Geometry: final body of the model. Coordinates: model frame, mm. A direction names the side the tool comes from. Round coordinates to 2 decimals unless told otherwise and drop trailing zeros. Loops run counter-clockwise (first coordinate to the right, second up) from the corner with the lowest first, then second, coordinate; pieces in that order, holes last. Notation, with made-up numbers: M -8.5,43.25 L 1.5,43.25 A27 ccw 1.5,75.25 Z; hole C 69,4.25 d5. An arc over 180 degrees is marked long. Return JSON: item names as keys, results as strings.
from build123d import *

# Parameters (mm, degrees)
BASPROSKE_W         = 5
BASPROSKE_H         = 11
TOOTHCUT_DEPTH      = 17.340134638
TEETHCUTS_COUNT     = 20
BORSKE_R            = 1.5
BORE_DEPTH          = 50.0000508
SKETCH_1_R          = 6
EXTRUDE_1_DEPTH     = 6
CUT_EXTRUDE_1_DEPTH = 14
SKETCH_3_R          = 2.7
CUT_EXTRUDE_2_DEPTH = 3


with BuildPart() as part:
    # BasProSke → Base-Revolve (revolve)
    with BuildSketch(Plane(origin=(0, 0, 0), x_dir=(1, 0, 0), z_dir=(0, 1, 0)), mode=Mode.PRIVATE) as base_revolve_sk:
        with Locations((2.5, 5.5)):
            Rectangle(BASPROSKE_W, BASPROSKE_H)
    revolve(base_revolve_sk.sketch.rotate(Axis((-10, 0, 0), (1, 0, 0)), 180), axis=Axis((-10, 0, 0), (1, 0, 0)))

    # TooCutSke → ToothCut (cut, through all)
    with BuildSketch(Plane(origin=(0, 0, 0), x_dir=(0, 0, -1), z_dir=(1, 0, 0))):
        with BuildLine():
            ThreePointArc((0.499924007, 8.734705318), (0, 8.749), (-0.499924007, 8.734705318))
            ThreePointArc((-0.499924007, 8.734705318), (-0.824302243, 9.905497836), (-1.485192705, 10.924909509))
            ThreePointArc((-1.485192705, 10.924909509), (0, 11.0254), (1.485192705, 10.924909509))
            ThreePointArc((1.485192705, 10.924909509), (0.824302243, 9.905497836), (0.499924007, 8.734705318))
        make_face()
    toothcut = extrude(amount=TOOTHCUT_DEPTH, mode=Mode.SUBTRACT)

    # TeethCuts: ToothCut ×20 about axis
    teethcuts_axis = Axis((0, 0, 0), (1, 0, 0))
    for i in range(1, TEETHCUTS_COUNT):
        add(toothcut.rotate(teethcuts_axis, i * 360 / TEETHCUTS_COUNT), mode=Mode.SUBTRACT)

    # BorSke → Bore (cut, symmetric)
    with BuildSketch(Plane(origin=(0, 0, 0), x_dir=(0, 0, -1), z_dir=(1, 0, 0))):
        with Locations(Location((0, 0, 0), (0, 0, 180))):
            Circle(BORSKE_R)
    extrude(amount=BORE_DEPTH, both=True, mode=Mode.SUBTRACT)

    # 草图1 → 凸台-拉伸1 (add)
    with BuildSketch(Plane(origin=(5, 0, 0), x_dir=(0, 0, -1), z_dir=(1, 0, 0))):
        with Locations(Location((0, 0, 0), (0, 0, 180))):
            Circle(SKETCH_1_R)
    extrude(amount=EXTRUDE_1_DEPTH)

    # 草图2 → 切除-拉伸1 (cut)
    with BuildSketch(Plane(origin=(11, 0, 0), x_dir=(0, 0, -1), z_dir=(1, 0, 0))):
        with BuildLine():
            Line((2.2, 1.565247584), (2.2, -1.565247584))
            ThreePointArc((2.2, -1.565247584), (-2.7, 0), (2.2, 1.565247584))
        make_face()
    extrude(amount=-CUT_EXTRUDE_1_DEPTH, mode=Mode.SUBTRACT)

    # 草图3 → 切除-拉伸2 (cut)
    with BuildSketch(Plane(origin=(11, 0, 0), x_dir=(0, 0, -1), z_dir=(1, 0, 0))):
        Circle(SKETCH_3_R)
    extrude(amount=-CUT_EXTRUDE_2_DEPTH, mode=Mode.SUBTRACT)


solid = part.part
Q1. Pin query (flat end, axial travel): pin 1 (1.6 mm diameter, centred on x = 5, y = 0, fed in from +Z); pin 2 (2 mm diameter, centred on x = 3.5, y = 8.5, fed in from +Z); pin 3 (1.5 mm diameter, centred on y = 7, z = 5.5, fed in from +X). Return the tip coordinate at first contact, or that it passes through.
Determined:
{"pin 1": "stops at z = 9.85", "pin 2": "stops at z = 7.96", "pin 3": "stops at x = 5"}
Q2. Reachability of faces 1 (the cylindrical face through (2.46, 3.85, 9.17)), 2 (the cylindrical face through (2.46, 8.47, -5.15)), 3 (the cylindrical face through (2.46, -3.85, -9.17)), 4 (the cylindrical face through (2.46, -7.53, 6.49)) from +Z, -Z, +X, -X, +Y, -Y: full face, straight path, thin tool, end or side. Return the list, or none.
Determined:
{"face 1": "+Z, +X, -X", "face 2": "+X, -X", "face 3": "-Z, +X, -X", "face 4": "+X, -X, -Y"}
Q3. Section query A-A (y = 0). Output: boundary loops of the cut face in (x, z), plus the area to 3 significant figures.
Determined:
{"outline": "M 0,-8.75 L 5,-8.75 L 5,-6 L 11,-6 L 11,-2.7 L 8,-2.7 L 8,-2.2 L 0,-2.2 Z; M 0,2.7 L 11,2.7 L 11,6 L 5,6 L 5,8.75 L 0,8.75 Z", "area": "104 mm^2"}
Q4. Pull-direction query (Z, two-part tool) for faces 5 (the cylindrical face through (2.465, -8.5, -5.156)), 6 (the cylindrical face through (7.958, -1.802, 5.723)), 7 (the cylindrical face through (2.465, 0.811, -9.876)); classes: pulls with the +Z half, pulls with the -Z half, needs draft (parallel to the pull), parting line crosses it, or undercut.
Determined:
{"face 5": "undercut", "face 6": "parting line crosses it", "face 7": "pulls with the -Z half"}
Q5. Section query B-B (z = 0). Output: boundary loops of the cut face in (x, y), plus the area to 3 significant figures.
Determined:
{"outline": "M 0,-8.75 L 5,-8.75 L 5,-6 L 11,-6 L 11,-2.7 L 0,-2.7 Z; M 0,2.7 L 11,2.7 L 11,6 L 5,6 L 5,8.75 L 0,8.75 Z", "area": "100 mm^2"}
Q6. Material intervals for L1, parallel to Z at x = 4.75, y = 0; L2, parallel to Y at x = 7, z = 0; L3, parallel to X at y = -2.75, z = -6.25, sorted ascending.
Determined:
{"L1": "z = -8.75 to -2.2, 2.7 to 8.75", "L2": "y = -6 to -2.7, 2.7 to 6", "L3": "x = 0 to 5"}
Q7. Section query D-D (y = -3.5). Output: boundary loops of the cut face in (x, z), plus the area to 3 significant figures.
Determined:
{"outline": "M 0,-8.73 L 5,-8.73 L 5,-4.87 L 11,-4.87 L 11,4.87 L 5,4.87 L 5,8.73 L 0,8.73 Z", "area": "146 mm^2"}
Q8. Section query C-C (x = 8.75). Output: boundary loops of the cut face in (y, z), plus the area to 3 significant figures.
Determined:
{"outline": "C 0,0 d12; hole C 0,0 d5.4", "area": "90.2 mm^2"}
